Build history of the part. All positions in model axes, mm. A direction names the side the tool comes from. Round coordinates to 2 decimals unless told otherwise and drop trailing zeros. Order: outer loops, then holes, each group sorted by start corner. A loop starts at its lowest first (then second) coordinate and runs counter-clockwise, first axis right, second up. Notation, with made-up numbers: (20.25, 76) -> (33.25, 76) arc R30 cw to (33.25, 101) -> close; hole circle Ø9 at (57, 5). An arc over 180 degrees is marked (long way). Use a Markdown table: item, result. Add a question column.
Item 1: 3-axis set-ups, long thin cutter, end or side, ignore diameter. For faces 1 (the face through (4, 16.224, -47)), 2 (the face through (4.22, 42.5, -40.54)), 3 (the face through (3.1, 12.7, -41.032)): which of +Z, -Z, +X, -X, +Y, -Y reach the whole face in a straight line?
Item 2: Slice it at C-C, the plane y = 53.5. Give the cut face in (x, z).
Item 3: Probe L1, parallel to Z at x = 3.5, y = 15.5; L2, parallel to Y at x = 7, z = -43; L3, parallel to Z at x = 3, y = 26. List the from-to ranges inside material, lowest first.
Item 4: Slice it at D-D, the plane x = 4. State how many separate pieces and enclosed holes the cut face has, plus the area to 3 significant figures.
Item 5: Slice it at B-B, the plane y = 32.5. Give the cut face in (x, z), plus the area to 3 significant figures.
Item 6: Pin check, flat tips, straight feed: pin 1 (2.5 mm diameter, centred on y = 24.97, z = -10.03, fed in from -X); pin 2 (4 mm diameter, centred on x = 2.5, y = 43, fed in from -Z); pin 3 (1 mm diameter, centred on x = 4, y = 43.5, fed in from -Z); pin 4 (4.5 mm diameter, centred on x = 5.5, y = 38, fed in from -Z). Stop position of each tip, or through.
Item 7: Slice it at A-A, the plane z = -24.5. Give the cut face in (x, y).
Item 8: Two-plate mould, pull along Y, no slides. Class faces 4 (the face through (4, 29, -60.532)), 5 (the face through (3.9, 5.9, -52.2)), 6 (the face through (3.944, 57.366, -41.919)): released by +Y, released by -Y, zero draft, split by the parting line, or undercut.
from build123d import *

# Parameters (mm, degrees)
SKETCH1_R      = 1.65
SKETCH1_R_2    = 1.75
EXTRUDE1_DEPTH = 8
SKETCH2_R      = 1
EXTRUDE2_DEPTH = 1
SKETCH3_R      = 1
EXTRUDE3_DEPTH = 1
SKETCH4_R      = 11.25
EXTRUDE4_DEPTH = 10


with BuildPart() as part:
    # Sketch1 → Extrude1 (new body)
    with BuildSketch(Plane(origin=(0, 0, 0), x_dir=(0, 0, -1), z_dir=(1, 0, 0))):
        with BuildLine():
            Line((53.032288553, 11.724414772), (53.032288553, 7.974414772))
            ThreePointArc((53.032288553, 7.974414772), (52.153608896, 5.853094429), (50.032288553, 4.974414772))
            Line((50.032288553, 4.974414772), (8.032288553, 4.974414772))
            ThreePointArc((8.032288553, 4.974414772), (5.910968209, 5.853094429), (5.032288553, 7.974414772))
            Line((5.032288553, 7.974414772), (5.032288553, 57.974414772))
            ThreePointArc((5.032288553, 57.974414772), (5.910968209, 60.095735116), (8.032288553, 60.974414772))
            Line((8.032288553, 60.974414772), (50.032288553, 60.974414772))
            ThreePointArc((50.032288553, 60.974414772), (52.153608896, 60.095735116), (53.032288553, 57.974414772))
            Line((53.032288553, 57.974414772), (53.032288553, 45.224414772))
            Line((53.032288553, 45.224414772), (48.532288553, 45.224414772))
            Line((48.532288553, 45.224414772), (48.532288553, 46.224414772))
            Line((48.532288553, 46.224414772), (46.032288553, 46.224414772))
            Line((46.032288553, 46.224414772), (46.032288553, 45.224414772))
            Line((46.032288553, 45.224414772), (41.032288553, 45.224414772))
            Line((41.032288553, 45.224414772), (41.032288553, 41.724414772))
            Line((41.032288553, 41.724414772), (46.032288553, 41.724414772))
            Line((46.032288553, 41.724414772), (46.032288553, 40.724414772))
            Line((46.032288553, 40.724414772), (48.532288553, 40.724414772))
            Line((48.532288553, 40.724414772), (48.532288553, 41.724414772))
            Line((48.532288553, 41.724414772), (53.032288553, 41.724414772))
            Line((53.032288553, 41.724414772), (53.032288553, 35.974414772))
            Line((53.032288553, 35.974414772), (59.532288553, 35.974414772))
            Line((59.532288553, 35.974414772), (60.532288553, 34.974414772))
            Line((60.532288553, 34.974414772), (60.532288553, 21.974414772))
            Line((60.532288553, 21.974414772), (59.532288553, 20.974414772))
            Line((59.532288553, 20.974414772), (53.032288553, 20.974414772))
            Line((53.032288553, 20.974414772), (53.032288553, 15.224414772))
            Line((53.032288553, 15.224414772), (48.532288553, 15.224414772))
            Line((48.532288553, 15.224414772), (48.532288553, 16.224414772))
            Line((48.532288553, 16.224414772), (46.032288553, 16.224414772))
            Line((46.032288553, 16.224414772), (46.032288553, 15.224414772))
            Line((46.032288553, 15.224414772), (41.032288553, 15.224414772))
            Line((41.032288553, 15.224414772), (41.032288553, 11.724414772))
            Line((41.032288553, 11.724414772), (46.032288553, 11.724414772))
            Line((46.032288553, 11.724414772), (46.032288553, 10.724414772))
            Line((46.032288553, 10.724414772), (48.532288553, 10.724414772))
            Line((48.532288553, 10.724414772), (48.532288553, 11.724414772))
            Line((48.532288553, 11.724414772), (53.032288553, 11.724414772))
        make_face()
        with Locations((41.032288553, 55.974414772)):
            Circle(SKETCH1_R, mode=Mode.SUBTRACT)
        with Locations((10.032288553, 55.974414772)):
            Circle(SKETCH1_R, mode=Mode.SUBTRACT)
        with Locations((41.032288553, 24.974414772)):
            Circle(SKETCH1_R, mode=Mode.SUBTRACT)
        with Locations((10.032288553, 24.974414772)):
            Circle(SKETCH1_R, mode=Mode.SUBTRACT)
        with Locations((52.032288553, 28.474414772)):
            Circle(SKETCH1_R_2, mode=Mode.SUBTRACT)
        with BuildLine():
            Line((22.032288553, 18.974414772), (22.032288553, 13.974414772))
            ThreePointArc((22.032288553, 13.974414772), (27.532288553, 8.474414772), (33.032288553, 13.974414772))
            Line((33.032288553, 13.974414772), (33.032288553, 18.974414772))
            ThreePointArc((33.032288553, 18.974414772), (27.532288553, 24.474414772), (22.032288553, 18.974414772))
        make_face(mode=Mode.SUBTRACT)
    extrude(amount=EXTRUDE1_DEPTH)

    # Sketch2 → Extrude2 (cut)
    with BuildSketch(Plane(origin=(0, 0, -41.032288553), x_dir=(-1, 0, 0), z_dir=(0, 0, -1))):
        with Locations((-4, 43.474414772)):
            Circle(SKETCH2_R)
    extrude(amount=-EXTRUDE2_DEPTH, mode=Mode.SUBTRACT)

    # Sketch3 → Extrude3 (cut)
    with BuildSketch(Plane(origin=(0, 0, -41.032288553), x_dir=(-1, 0, 0), z_dir=(0, 0, -1))):
        with Locations((-4, 13.474414772)):
            Circle(SKETCH3_R)
    extrude(amount=-EXTRUDE3_DEPTH, mode=Mode.SUBTRACT)

    # Sketch4 → Extrude4 (cut)
    with BuildSketch(Plane(origin=(8, 0, 0), x_dir=(0, 0, -1), z_dir=(1, 0, 0))):
        with Locations((25.532288553, 40.474414772)):
            Circle(SKETCH4_R)
    extrude(amount=-EXTRUDE4_DEPTH, mode=Mode.SUBTRACT)


solid = part.part
Check sheet entries:
| question | item | result |
|---|---|---|
| 1 | face 1 | +X, -X |
| 1 | face 2 | -Z |
| 1 | face 3 | -Z, +X, -X |
| 2 | outline | (0, -53.03) -> (8, -53.03) -> (8, -5.03) -> (0, -5.03) -> close |
| 3 | L1 | -53.03 to -48.53, -46.03 to -33.03, -22.03 to -5.03 |
| 3 | L2 | 4.97 to 11.72, 15.22 to 41.72, 45.22 to 60.97 |
| 3 | L3 | -60.53 to -42.32, -39.74 to -11.32, -8.74 to -5.03 |
| 4 | separate pieces | 1 |
| 4 | enclosed holes | 7 |
| 4 | area | 2,100 mm2 |
| 5 | outline | (0, -60.53) -> (8, -60.53) -> (8, -33.47) -> (0, -33.47) -> close; (0, -17.6) -> (8, -17.6) -> (8, -5.03) -> (0, -5.03) -> close |
| 5 | area | 317 mm2 |
| 6 | pin 1 | through |
| 6 | pin 2 | z = -53.03 |
| 6 | pin 3 | z = -40.03 |
| 6 | pin 4 | z = -59.76 |
| 7 | outline | (0, 4.97) -> (8, 4.97) -> (8, 9.39) -> (0, 9.39) -> close; (0, 23.56) -> (8, 23.56) -> (8, 29.27) -> (0, 29.27) -> close; (0, 51.68) -> (8, 51.68) -> (8, 60.97) -> (0, 60.97) -> close |
| 8 | face 4 | zero draft |
| 8 | face 5 | released by -Y |
| 8 | face 6 | undercut |
